from build123d import *

# Parameters (mm, degrees)
SKETCH1_W                       = 45
SKETCH1_H                       = 200
BOSS_EXTRUDE1_DEPTH             = 735
FILLET1_R                       = 4
F_6_0MM_DOWEL_SLOT1_D           = 6
F_6_0MM_DOWEL_SLOT1_DEPTH       = 63.197418143
F_6_0MM_DOWEL_SLOT1_CSINK_D     = 6.05
F_6_0MM_DOWEL_SLOT1_CSINK_ANGLE = 90
F_6_0MM_DOWEL_SLOT1_TIP         = 1.802581857
F_6_0MM_DOWEL_SLOT2_D           = 6
F_6_0MM_DOWEL_SLOT2_DEPTH       = 63.197418143
F_6_0MM_DOWEL_SLOT2_CSINK_D     = 6.05
F_6_0MM_DOWEL_SLOT2_CSINK_ANGLE = 90
F_6_0MM_DOWEL_SLOT2_TIP         = 1.802581857
F_6_0MM_DOWEL_SLOT6_D           = 6
F_6_0MM_DOWEL_SLOT6_DEPTH       = 28.197418143
F_6_0MM_DOWEL_SLOT6_CSINK_D     = 6.05
F_6_0MM_DOWEL_SLOT6_CSINK_ANGLE = 90
F_6_0MM_DOWEL_SLOT6_TIP         = 1.802581857


with BuildPart() as part:
    # Sketch1 → Boss-Extrude1 (new body)
    with BuildSketch(Plane.XY):
        with Locations((-8.688255411, 34.272684877)):
            Rectangle(SKETCH1_W, SKETCH1_H)
    extrude(amount=BOSS_EXTRUDE1_DEPTH)

    # Fillet1
    fillet1_edges = [part.edges().sort_by_distance(p)[0] for p in [
        (13.811744589, 134.272684877, 367.5),
        (13.811744589, -65.727315123, 367.5),
        (-31.188255411, -65.727315123, 367.5),
        (-31.188255411, 134.272684877, 367.5),
    ]]
    fillet(fillet1_edges, radius=FILLET1_R)

    # Ø6.0mm Dowel Slot1
    with Locations(Plane(origin=(863.811744589, -65.727315123, 780), x_dir=(1, 0, 0), z_dir=(0, 0, 1))):
        with Locations((-872.5, 160), (-872.5, 100), (-872.5, 40)):
            CounterSinkHole(F_6_0MM_DOWEL_SLOT1_D / 2, F_6_0MM_DOWEL_SLOT1_CSINK_D / 2, depth=F_6_0MM_DOWEL_SLOT1_DEPTH, counter_sink_angle=F_6_0MM_DOWEL_SLOT1_CSINK_ANGLE)
            with Locations((0, 0, -(F_6_0MM_DOWEL_SLOT1_DEPTH + F_6_0MM_DOWEL_SLOT1_TIP / 2))):  # 118° drill point
                Cone(0, F_6_0MM_DOWEL_SLOT1_D / 2, F_6_0MM_DOWEL_SLOT1_TIP, mode=Mode.SUBTRACT)

    # Ø6.0mm Dowel Slot2
    with Locations(Plane(origin=(863.811744589, -65.727315123, -45), x_dir=(-1, 0, 0), z_dir=(0, 0, -1))):
        with Locations((872.5, 160), (872.5, 100), (872.5, 40)):
            CounterSinkHole(F_6_0MM_DOWEL_SLOT2_D / 2, F_6_0MM_DOWEL_SLOT2_CSINK_D / 2, depth=F_6_0MM_DOWEL_SLOT2_DEPTH, counter_sink_angle=F_6_0MM_DOWEL_SLOT2_CSINK_ANGLE)
            with Locations((0, 0, -(F_6_0MM_DOWEL_SLOT2_DEPTH + F_6_0MM_DOWEL_SLOT2_TIP / 2))):  # 118° drill point
                Cone(0, F_6_0MM_DOWEL_SLOT2_D / 2, F_6_0MM_DOWEL_SLOT2_TIP, mode=Mode.SUBTRACT)

    # Ø6.0mm Dowel Slot6
    with Locations(Plane(origin=(863.811744589, 146.272684877, -45), x_dir=(0, 0, 1), z_dir=(0, 1, 0))):
        with Locations((22.5, 1726.5), (22.5, 1640.5), (802.5, 1726.5), (802.5, 1640.5), (22.5, -955.960621131), (22.5, -1636.5), (802.5, -1462.5), (802.5, -1636.5), (22.5, -1722.5), (802.5, -1722.5), (22.5, -1550.5), (802.5, -640.31), (120, -1722.5), (217.5, -1722.5), (315, -1722.5), (412.5, -1722.5), (510, -1722.5), (607.5, -1722.5), (705, -1722.5), (22.5, -861.25), (22.5, -883.75), (-22.496198074, -917.60220409), (802.5, -861.25), (802.5, -883.75), (847.496198074, -917.60220409), (802.5, -529.84), (22.5, -750.249617159), (-341.005231297, -650.318686522), (1166.005231297, -650.318686522), (-310.084924074, 22.5), (-310.084924074, 67.5), (22.5, 67.5), (22.5, 22.5), (802.5, 67.5), (802.5, 22.5), (1133.730020848, 67.5), (1133.730020848, 22.5), (1166.005231297, 740.318686522), (802.560751791, 973.75), (802.560751791, 951.25), (847.496198074, 1007.60220409), (-22.496198074, 1007.60220409), (22.560751791, 951.25), (-341.005231297, 740.318686522), (22.5, 1812.5), (802.5, 1812.5), (22.5, 1552.5), (802.5, 1552.5), (-102.162023695, -850.748960129), (-181.827849315, -783.895716167), (-261.493674936, -717.042472206), (927.162023695, -850.748960129), (1006.827849315, -783.895716167), (1086.493674936, -717.042472206), (1086.493674936, 807.042472206), (1006.827849315, 873.895716167), (927.162023695, 940.748960129), (-102.162023695, 940.748960129), (-181.827849315, 873.895716167), (-261.493674936, 807.042472206), (-199.224924074, 67.5), (-88.364924074, 67.5), (-199.224924074, 22.5), (-88.364924074, 22.5), (912.010020848, 67.5), (1022.870020848, 67.5), (912.010020848, 22.5), (1022.870020848, 22.5), (120, 67.5), (217.5, 67.5), (315, 67.5), (607.5, 67.5), (705, 67.5), (510, 67.5), (120, 22.5), (217.5, 22.5), (315, 22.5), (510, 22.5), (607.5, 22.5), (705, 22.5), (412.5, 22.5), (22.5, -750.78), (22.5, -640.31), (22.5, -529.84), (22.5, -419.37), (22.5, -308.9), (22.5, -198.43), (22.5, -87.96), (802.5, -750.78), (802.5, -419.37), (802.5, -308.9), (802.5, -198.43), (22.5, 177.97), (22.5, 288.44), (22.5, 398.91), (22.5, 509.38), (22.5, 619.85), (22.5, 730.32), (22.5, 840.79), (802.5, -87.96), (802.5, 177.97), (802.5, 288.44), (120.000330201, 1812.753749877), (217.5, 1812.5), (315, 1812.5), (412.5, 1812.5), (510, 1812.5), (607.5, 1812.5), (705, 1812.5), (120.060751791, 951.25), (217.560751791, 951.25), (315.060751791, 951.25), (412.560751791, 951.25), (510.060751791, 951.25), (607.560751791, 951.25), (705.060751791, 951.25), (656.310751791, 973.75), (558.810751791, 973.75), (461.310751791, 973.75), (363.810751791, 973.75), (266.310751791, 973.75), (168.810751791, 973.75), (120, -861.25), (217.5, -861.25), (315, -861.25), (412.5, -861.25), (510, -861.25), (607.5, -861.25), (705, -861.25), (656.25, -883.75), (558.75, -883.75), (461.25, -883.75), (168.75, -883.75), (266.25, -883.75), (363.75, -883.75), (802.560751791, -955.960621131), (412.5, 67.5), (802.5, 730.32), (802.560751791, 840.79), (802.5, 398.91), (802.5, 509.38), (802.5, 619.85), (-360.000025903, 699.425529794), (-360.000025903, -609.521258848), (-360.000025903, 598.725529794), (-360.000025903, 498.025529794), (-360.000025903, 397.325529794), (-360.000025903, 296.625529794), (-360.000025903, 195.925529794), (-360.000025903, 95.225529794), (-360.000025903, -5.474470206), (-360.000025903, -106.174470206), (-360.000025903, -206.874470206), (-360.000025903, -307.574470206), (-360.000025903, -408.274470206), (-360.000025903, -508.974470206), (1185.00101945, 699.425529452), (1185.000941829, 598.725529794), (1185.000864209, 498.025529794), (1185.000708968, 296.625529794), (1185.000631348, 195.925529794), (1185.000553727, 95.225529794), (1185.000476107, -5.474470206), (1185.000398486, -106.174470206), (1185.000320866, -206.874470206), (1185.000165625, -408.274470206), (1185.000088004, -508.974470206), (1185.000786589, 397.325529794), (22.560751791, 1016.385842825), (802.560751791, 1016.385842825), (802.560751791, -1550.5), (22.560751791, 973.75), (802.560751791, -363.966698641)):
            CounterSinkHole(F_6_0MM_DOWEL_SLOT6_D / 2, F_6_0MM_DOWEL_SLOT6_CSINK_D / 2, depth=F_6_0MM_DOWEL_SLOT6_DEPTH, counter_sink_angle=F_6_0MM_DOWEL_SLOT6_CSINK_ANGLE)
            with Locations((0, 0, -(F_6_0MM_DOWEL_SLOT6_DEPTH + F_6_0MM_DOWEL_SLOT6_TIP / 2))):  # 118° drill point
                Cone(0, F_6_0MM_DOWEL_SLOT6_D / 2, F_6_0MM_DOWEL_SLOT6_TIP, mode=Mode.SUBTRACT)


solid = part.part
Design review of the part built by this model. Coordinates are the model's own, in mm. Coordinates: 2 decimals unless noted, no trailing zeros. Use one line per item in the form item = value. Start each with the question number.
(1) The part is to be moulded in two halves that separate along Y. For faces 1 (the flat face through (-9, -65.727, 362)), 2 (the flat face through (-9, 134.273, 362)), 3 (the flat face through (-31.188, 33, 362)), say which applies: +Y half, -Y half, draft (parallel to the pull), parting line (faces both ways), or undercut.
(2) For probe 1 along X at (y, z) = (122.5, 270); probe 2 along X at (y, z) = (121.5, 221.25); probe 3 along Y at (x, z) = (12, 410), list the stretches that pass through material, from the lowest coordinate up.
(3) Insertion check: pin 1 (3.5 mm diameter, centred on x = 2.56, z = 75, fed in from +Y); pin 2 (5 mm diameter, centred on x = -8.69, y = 34.27, fed in from -Z); pin 3 (5 mm diameter, centred on x = -19.94, z = 318.75, fed in from +Y). Each pin has a flat end and moves straight along its axis. Give the tip position at first contact, or say it passes through.
Answer block:
q1.face_1 = -Y half
q1.face_2 = +Y half
q1.face_3 = draft
q2.probe_1 = -31.19 to -0.44, 5.56 to 13.81
q2.probe_2 = -31.19 to -22.94, -16.94 to 13.81
q2.probe_3 = -65.08 to 133.62
q3.pin_1 = 117.33
q3.pin_2 = 18.5
q3.pin_3 = 117.78
